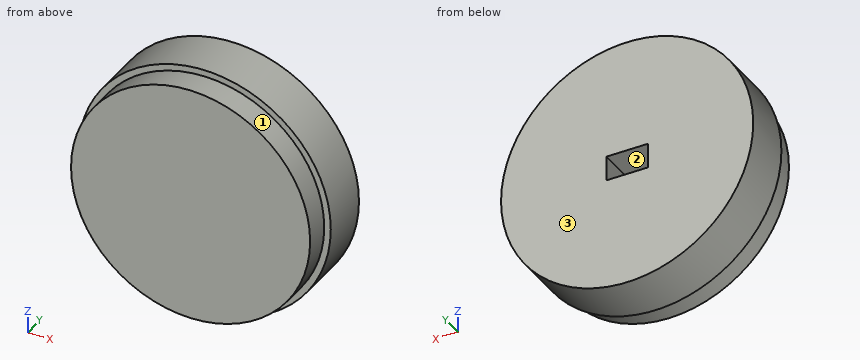
```python
from build123d import *

# Parameters (mm, degrees)
SKETCH1_R           = 15
BOSS_EXTRUDE1_DEPTH = 9
SKETCH6_OUTSIDE_W   = 40.674
SKETCH6_OUTSIDE_H   = 40.674
SKETCH6_OUTSIDE_R   = 14.222015383
CUT_EXTRUDE4_DEPTH  = 3
SKETCH8_W           = 4.952506836
SKETCH8_H           = 2.956951794
CUT_EXTRUDE5_DEPTH  = 6


with BuildPart() as part:
    # Sketch1 → Boss-Extrude1 (new body)
    with BuildSketch(Plane(origin=(0, 0, 0), x_dir=(1, 0, 0), z_dir=(0, 1, 0))):
        Circle(SKETCH1_R)
    extrude(amount=BOSS_EXTRUDE1_DEPTH)

    # Sketch6 outside → Cut-Extrude4 (cut)
    with BuildSketch(Plane.XZ):
        Rectangle(SKETCH6_OUTSIDE_W, SKETCH6_OUTSIDE_H)
        Circle(SKETCH6_OUTSIDE_R, mode=Mode.SUBTRACT)
    extrude(amount=-CUT_EXTRUDE4_DEPTH, mode=Mode.SUBTRACT)

    # Sketch8 → Cut-Extrude5 (cut)
    with BuildSketch(Plane(origin=(0, 9, 0), x_dir=(1, 0, 0), z_dir=(0, 1, 0))):
        with Locations((0, -0.017356659)):
            Rectangle(SKETCH8_W, SKETCH8_H)
    extrude(amount=-CUT_EXTRUDE5_DEPTH, mode=Mode.SUBTRACT)


solid = part.part
```
Verification items for the finished model (mm, model axes). Face numbers are marked on the shaded views. A direction names the side the tool comes from. Round coordinates to 2 decimals unless told otherwise and drop trailing zeros. Write each loop counter-clockwise with the first axis right and the second up, starting at its lowest first coordinate (ties: lowest second). Pieces come first, ordered by that corner, then holes. Notation, with made-up numbers: (47, 4.25) - (64, 4.25) arc R24 cw to (64, 26.25) - close; hole circle Ø1 at (-9.5, -38). An arc over 180 degrees is marked (long way). Answer as a JSON object with one key per item and string values. Group by question number.
Q1. Section check C-C, the plane z = 13. Enter the section's corners in (x, y), plus the area to 3 significant figures.
Q2. Thickness scan on line 1 (X direction, y = 8.75, z = 0); line 2 (Z direction, x = -1, y = 7.25); line 3 (Z direction, x = -2.25, y = 4). Record the ranges inside material, lowest first.
Q3. Section check D-D, the plane y = 1.5. Enter the section's corners in (x, z).
Q4. Tool access check on the marked faces 1, 2 and 3. Record the directions out of +Z, -Z, +X, -X, +Y, -Y that give a thin tool (end or side, any length) a straight path to the whole face; none if there is none.
Q5. Go/stop test with flat-tipped pins: pin 1 Ø1.5 at (x, z) = (0, 0.5) entering from +Y; pin 2 Ø1.5 at (x, y) = (-1, 6.5) entering from +Z. Record where each tip stops, or that it passes through.
Q6. Section check B-B, the plane x = 0. Enter the section's corners in (y, z).
Q7. Section check A-A, the plane y = 7. Enter the section's corners in (x, z), plus the area to 3 significant figures.
Found:
{
 "1": {"outline": "(-7.48, 3) - (-5.77, 3) - (-5.77, 0) - (5.77, 0) - (5.77, 3) - (7.48, 3) - (7.48, 9) - (-7.48, 9) - close", "area": "124 mm^2"},
 "2": {"line 1": "x = -15 to -2.48, 2.48 to 15", "line 2": "z = -14.97 to -1.46, 1.5 to 14.97", "line 3": "z = -14.83 to -1.46, 1.5 to 14.83"},
 "3": {"outline": "circle Ø28.44 at (0, 0)"},
 "4": {"face 1": "-Y", "face 2": "+Y", "face 3": "+Z, -Z, +X, -X, +Y"},
 "5": {"pin 1": "stops at y = 3", "pin 2": "stops at z = 15"},
 "6": {"outline": "(0, -14.22) - (3, -14.22) - (3, -15) - (9, -15) - (9, -1.46) - (3, -1.46) - (3, 1.5) - (9, 1.5) - (9, 15) - (3, 15) - (3, 14.22) - (0, 14.22) - close"},
 "7": {"outline": "circle Ø30 at (0, 0); hole (-2.48, -1.46) - (2.48, -1.46) - (2.48, 1.5) - (-2.48, 1.5) - close", "area": "692 mm^2"}
}
